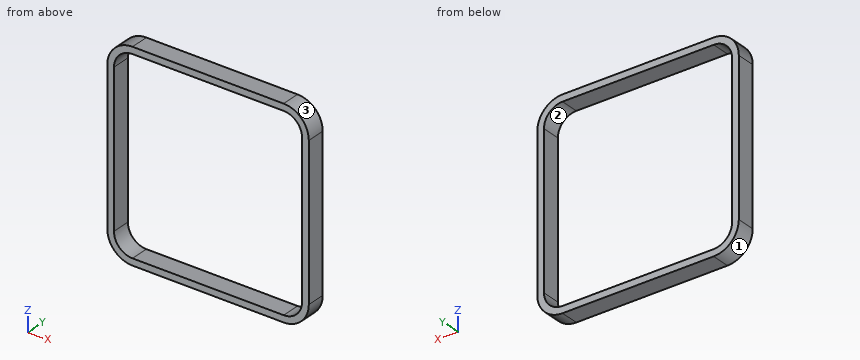
```python
from build123d import *

# Parameters (mm, degrees)
BOSS_EXTRUDE1_DEPTH = 150
CUT_EXTRUDE1_DEPTH  = 110
SKETCH3_R           = 52.074473314
CUT_EXTRUDE2_DEPTH  = 110
CUT_EXTRUDE4_DEPTH  = 40


with BuildPart() as part:
    # Sketch1 → Boss-Extrude1 (new body)
    with BuildSketch(Plane(origin=(0, 0, 0), x_dir=(1, 0, 0), z_dir=(0, 1, 0))):
        with BuildLine():
            Line((-450, -600), (450, -600))
            ThreePointArc((450, -600), (556.066017178, -556.066017178), (600, -450))
            Line((600, -450), (600, 450))
            ThreePointArc((600, 450), (556.066017178, 556.066017178), (450, 600))
            Line((450, 600), (-450, 600))
            ThreePointArc((-450, 600), (-556.066017178, 556.066017178), (-600, 450))
            Line((-600, 450), (-600, -450))
            ThreePointArc((-600, -450), (-556.066017178, -556.066017178), (-450, -600))
        make_face()
    extrude(amount=BOSS_EXTRUDE1_DEPTH)

    # Sketch2 → Cut-Extrude1 (cut)
    with BuildSketch(Plane(origin=(0, 150, 0), x_dir=(1, 0, 0), z_dir=(0, 1, 0))):
        with BuildLine():
            Line((450, 560), (-450, 560))
            ThreePointArc((-450, 560), (-527.781745931, 527.781745931), (-560, 450))
            Line((-560, 450), (-560, -450))
            ThreePointArc((-560, -450), (-527.781745931, -527.781745931), (-450, -560))
            Line((-450, -560), (450, -560))
            ThreePointArc((450, -560), (527.781745931, -527.781745931), (560, -450))
            Line((560, -450), (560, 450))
            ThreePointArc((560, 450), (527.781745931, 527.781745931), (450, 560))
        make_face()
    extrude(amount=-CUT_EXTRUDE1_DEPTH, mode=Mode.SUBTRACT)

    # Sketch3 → Cut-Extrude2 (cut)
    with BuildSketch(Plane(origin=(0, 40, 0), x_dir=(1, 0, 0), z_dir=(0, 1, 0))):
        with Locations((249.348788186, 217.558417351)):
            Circle(SKETCH3_R)
    extrude(amount=-CUT_EXTRUDE2_DEPTH, mode=Mode.SUBTRACT)

    # Sketch7 → Cut-Extrude4 (cut)
    with BuildSketch(Plane.XZ):
        with BuildLine():
            Line((600, -450), (600, 450))
            ThreePointArc((600, 450), (556.066017178, 556.066017178), (450, 600))
            Line((450, 600), (-450, 600))
            ThreePointArc((-450, 600), (-556.066017178, 556.066017178), (-600, 450))
            Line((-600, 450), (-600, -450))
            ThreePointArc((-600, -450), (-556.066017178, -556.066017178), (-450, -600))
            Line((-450, -600), (450, -600))
            ThreePointArc((450, -600), (556.066017178, -556.066017178), (600, -450))
        make_face()
    extrude(amount=-CUT_EXTRUDE4_DEPTH, mode=Mode.SUBTRACT)


solid = part.part
```
Check sheet for the modelled part. Datum: model origin and axes. Units: mm. Face numbers are marked on the shaded views. Give positions to 0.01 mm unless a question says otherwise; leave off trailing zeros. Order: outer loops, then holes, each group sorted by start corner. A loop starts at its lowest first (then second) coordinate and runs counter-clockwise, first axis right, second up. Notation, with made-up numbers: (54.5, 45.5) -> (88.5, 45.5) arc R31 ccw to (88.5, 83.5) -> close; hole circle Ø11 at (86.25, -35.5). An arc over 180 degrees is marked (long way). Use CSV: the item, a comma, the result in double quotes. Start each with the question number.
1) Sectioned sample at C-C, the plane y = 116.5. Record the boundary of the cut face in (x, z).
2) Go/stop test with a flat-tipped pin: P1, Ø10, axis at y = 72.5, z = 473, coming from the -X side. Record where the tip stops, or that it passes through.
3) Material ranges on line 1 (Z direction, x = -412, y = 61.5); line 2 (X direction, y = 116, z = -505), recorded low to high. Write a range as from..to.
4) Sectioned sample at B-B, the plane z = -33.5. Record the boundary of the cut face in (x, y).
5) Sectioned sample at A-A, the plane x = 199. Record the boundary of the cut face in (y, z), plus the area to 3 significant figures.
6) Mould release check, pull along Z, two halves, no side actions. Record for the marked faces 1, 2 and 3: released by +Z, released by -Z, zero draft, split by the parting line, or undercut.
Recorded:
1,outline,"(-600, -450) arc R150 ccw to (-450, -600) -> (450, -600) arc R150 ccw to (600, -450) -> (600, 450) arc R150 ccw to (450, 600) -> (-450, 600) arc R150 ccw to (-600, 450) -> close; hole (-560, -450) arc R110 ccw to (-450, -560) -> (450, -560) arc R110 ccw to (560, -450) -> (560, 450) arc R110 ccw to (450, 560) -> (-450, 560) arc R110 ccw to (-560, 450) -> close"
2,P1,"x = -598.92"
3,line 1,"-600..-560, 560..600"
3,line 2,"-589.55..-545.26, 545.26..589.55"
4,outline,"(-600, 40) -> (-560, 40) -> (-560, 150) -> (-600, 150) -> close; (560, 40) -> (600, 40) -> (600, 150) -> (560, 150) -> close"
5,outline,"(40, -600) -> (150, -600) -> (150, -560) -> (40, -560) -> close; (40, 560) -> (150, 560) -> (150, 600) -> (40, 600) -> close"
5,area,"8,800 mm2"
6,face 1,"released by -Z"
6,face 2,"undercut"
6,face 3,"released by +Z"
